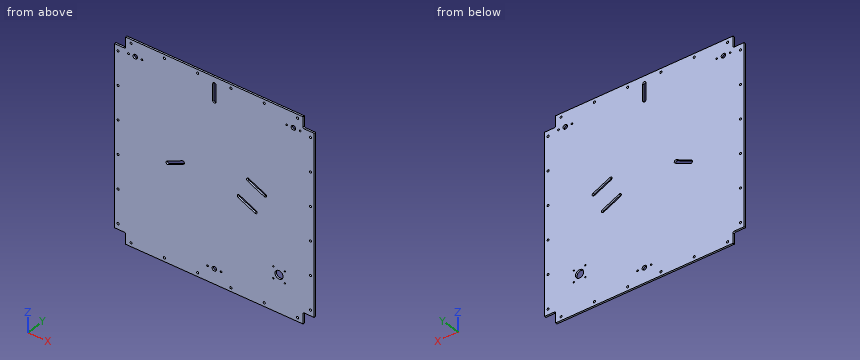
```python
from build123d import *

# Parameters (mm, degrees)
SKETCH2_W             = 540
SKETCH2_H             = 540
SKETCH2_R             = 6
SKETCH2_R_2           = 11
BOSS_EXTRUDE1_DEPTH   = 4.7625
M4_CLEARANCE_HOLE1_D  = 4.5
M3_CLEARANCE_HOLE10_D = 3.4
SKETCH5_W             = 30
SKETCH5_H             = 30
CUT_EXTRUDE1_DEPTH    = 764.6901737
FILLET1_R             = 3.175
CUT_EXTRUDE2_DEPTH    = 764.6901737
CUT_EXTRUDE3_DEPTH    = 764.6901737
M5_CLEARANCE_HOLE1_D  = 5.8
LPATTERN1_COUNT       = 6
LPATTERN1_PITCH       = 90
M5_CLEARANCE_HOLE2_D  = 5.8
LPATTERN2_COUNT       = 6
LPATTERN2_PITCH       = 90
M5_CLEARANCE_HOLE3_D  = 5.8
LPATTERN3_COUNT       = 6
LPATTERN3_PITCH       = 90
M5_CLEARANCE_HOLE4_D  = 5.8
LPATTERN4_COUNT       = 6
LPATTERN4_PITCH       = 90


with BuildPart() as part:
    # Sketch2 → Boss-Extrude1 (new body)
    with BuildSketch(Plane(origin=(0, 0, 0), x_dir=(1, 0, 0), z_dir=(0, 1, 0))):
        with Locations((270, 270)):
            Rectangle(SKETCH2_W, SKETCH2_H)
        with Locations(Location((56.175, 40, 0), (0, 0, 90))):
            Circle(SKETCH2_R, mode=Mode.SUBTRACT)
        with Locations(Location((483.825, 40, 0), (0, 0, 90))):
            Circle(SKETCH2_R, mode=Mode.SUBTRACT)
        with Locations(Location((270, 500, 0), (0, 0, 90))):
            Circle(SKETCH2_R, mode=Mode.SUBTRACT)
        with Locations(Location((445, 440, 0), (0, 0, 90))):
            Circle(SKETCH2_R_2, mode=Mode.SUBTRACT)
    extrude(amount=BOSS_EXTRUDE1_DEPTH)

    # M4 Clearance Hole1 (through all)
    with Locations(Plane(origin=(74.425, 4.7625, -40), x_dir=(0, 0, 1), z_dir=(0, 1, 0))):
        with Locations((0, 0), (0, -36.5), (-460, 177.325), (-460, 213.825), (0, 391.15), (0, 427.65)):
            Hole(M4_CLEARANCE_HOLE1_D / 2)

    # M3 Clearance Hole10 (through all)
    with Locations(Plane(origin=(429.5, 4.7625, -455.5), x_dir=(0, 0, 1), z_dir=(0, 1, 0))):
        with Locations((0, 0), (0, 31), (31, 31), (31, 0)):
            Hole(M3_CLEARANCE_HOLE10_D / 2)

    # Sketch5 → Cut-Extrude1 (cut, through all)
    with BuildSketch(Plane(origin=(0, 4.7625, 0), x_dir=(1, 0, 0), z_dir=(0, 1, 0))):
        with Locations((15, 15)):
            Rectangle(SKETCH5_W, SKETCH5_H)
        with Locations((525, 15)):
            Rectangle(SKETCH5_W, SKETCH5_H)
        with Locations((525, 525)):
            Rectangle(SKETCH5_W, SKETCH5_H)
        with Locations((15, 525)):
            Rectangle(SKETCH5_W, SKETCH5_H)
    extrude(amount=-CUT_EXTRUDE1_DEPTH, mode=Mode.SUBTRACT)

    # Fillet1
    fillet1_edges = [part.edges().sort_by_distance(p)[0] for p in [
        (510, 2.38125, -30),
        (510, 2.38125, -510),
        (30, 2.38125, -510),
        (30, 2.38125, -30),
    ]]
    fillet(fillet1_edges, radius=FILLET1_R)

    # Sketch6 → Cut-Extrude2 (cut, through all)
    with BuildSketch(Plane(origin=(0, 4.7625, 0), x_dir=(1, 0, 0), z_dir=(0, 1, 0))):
        with BuildLine():
            Line((379.893699129, 307.475094097), (334.552801834, 286.398969393))
            ThreePointArc((334.552801834, 286.398969393), (332.490296164, 280.753522523), (338.135743034, 278.691016853))
            Line((338.135743034, 278.691016853), (383.476640328, 299.767141557))
            ThreePointArc((383.476640328, 299.767141557), (385.539145999, 305.412588427), (379.893699129, 307.475094097))
        make_face()
        with BuildLine():
            Line((405.008613589, 253.445580936), (359.667716294, 232.369456232))
            ThreePointArc((359.667716294, 232.369456232), (357.605210624, 226.724009362), (363.250657494, 224.661503692))
            Line((363.250657494, 224.661503692), (408.591554788, 245.737628396))
            ThreePointArc((408.591554788, 245.737628396), (410.654060459, 251.383075266), (405.008613589, 253.445580936))
        make_face()
    extrude(amount=-CUT_EXTRUDE2_DEPTH, mode=Mode.SUBTRACT)

    # Sketch9 → Cut-Extrude3 (cut, through all)
    with BuildSketch(Plane(origin=(0, 4.7625, 0), x_dir=(1, 0, 0), z_dir=(0, 1, 0))):
        with BuildLine():
            Line((274.25, 19), (274.25, 64))
            ThreePointArc((274.25, 64), (270, 68.25), (265.75, 64))
            Line((265.75, 64), (265.75, 19))
            ThreePointArc((265.75, 19), (270, 14.75), (274.25, 19))
        make_face()
        with BuildLine():
            Line((186.642601301, 263.737436412), (145.835793736, 282.705948646))
            ThreePointArc((145.835793736, 282.705948646), (140.190346866, 280.643442976), (142.252852537, 274.997996106))
            Line((142.252852537, 274.997996106), (183.059660101, 256.029483872))
            ThreePointArc((183.059660101, 256.029483872), (188.705106971, 258.091989542), (186.642601301, 263.737436412))
        make_face()
    extrude(amount=-CUT_EXTRUDE3_DEPTH, mode=Mode.SUBTRACT)

    # M5 Clearance Hole1 (through all)
    with Locations(Plane(origin=(45, 4.7625, -10), x_dir=(0, 0, 1), z_dir=(0, 1, 0))):
        with Locations((0, 0)):
            m5_clearance_hole1 = Hole(M5_CLEARANCE_HOLE1_D / 2)

    # LPattern1: M5 Clearance Hole1 ×6
    with Locations(*[(i * LPATTERN1_PITCH, 0, 0) for i in range(1, LPATTERN1_COUNT)]):
        add(m5_clearance_hole1, mode=Mode.SUBTRACT)

    # M5 Clearance Hole2 (through all)
    with Locations(Plane(origin=(10, 4.7625, -495), x_dir=(0, 0, 1), z_dir=(0, 1, 0))):
        with Locations((0, 0)):
            m5_clearance_hole2 = Hole(M5_CLEARANCE_HOLE2_D / 2)

    # LPattern2: M5 Clearance Hole2 ×6
    with Locations(*[(0, 0, i * LPATTERN2_PITCH) for i in range(1, LPATTERN2_COUNT)]):
        add(m5_clearance_hole2, mode=Mode.SUBTRACT)

    # M5 Clearance Hole3 (through all)
    with Locations(Plane(origin=(495, 4.7625, -530), x_dir=(0, 0, 1), z_dir=(0, 1, 0))):
        with Locations((0, 0)):
            m5_clearance_hole3 = Hole(M5_CLEARANCE_HOLE3_D / 2)

    # LPattern3: M5 Clearance Hole3 ×6
    with Locations(*[(-i * LPATTERN3_PITCH, 0, 0) for i in range(1, LPATTERN3_COUNT)]):
        add(m5_clearance_hole3, mode=Mode.SUBTRACT)

    # M5 Clearance Hole4 (through all)
    with Locations(Plane(origin=(530, 4.7625, -45), x_dir=(0, 0, 1), z_dir=(0, 1, 0))):
        with Locations((0, 0)):
            m5_clearance_hole4 = Hole(M5_CLEARANCE_HOLE4_D / 2)

    # LPattern4: M5 Clearance Hole4 ×6
    with Locations(*[(0, 0, -i * LPATTERN4_PITCH) for i in range(1, LPATTERN4_COUNT)]):
        add(m5_clearance_hole4, mode=Mode.SUBTRACT)


solid = part.part
```
Read the model definition and answer for the solid it produces. Units are mm, in the model's axes. Coordinates: 2 decimals unless noted, no trailing zeros. Write each loop counter-clockwise with the first axis right and the second up, starting at its lowest first coordinate (ties: lowest second). Pieces come first, ordered by that corner, then holes. Notation, with made-up numbers: (84.5, 11.25) - (102.5, 11.25) arc R13 cw to (102.5, 20.25) - close; hole circle Ø11 at (19, 35.25). An arc over 180 degrees is marked (long way). Answer as a JSON object with one key per item and string values. Group by question number.
1. A cutting plane is placed at A-A (x = 166). Determine the outline of the cut face in (y, z), plus the area to 3 significant figures.
2. This flat-tipped pin is pushed along its axis until it touches: P1, Ø1.4, axis at x = 13.5, y = 1.5, coming from the -Z side. Where does it stop, or does it pass through?
3. Consider L1, parallel to X at y = 3.15, z = -315; L2, parallel to X at y = 3.65, z = -424.5; L3, parallel to Z at x = 405, y = 3.35. Determine where each line is inside the solid, lowest interval first. Write a range as [from, to].
4. A cutting plane is placed at B-B (y = 2.05). Give the number of separate pieces and of enclosed holes in the cut face, plus the area to 3 significant figures.
Worked out:
{
 "1": {"outline": "(0, -540) - (4.76, -540) - (4.76, -273.33) - (0, -273.33) - close; (0, -263.96) - (4.76, -263.96) - (4.76, 0) - (0, 0) - close", "area": "2,530 mm²"},
 "2": {"P1": "stops at z = -510"},
 "3": {"L1": "x = [0, 7.1], [12.9, 527.1], [532.9, 540]", "L2": "x = [0, 427.8], [431.2, 458.8], [462.2, 540]", "L3": "z = [-540, -532.9], [-527.1, -253.44], [-244.07, -12.9], [-7.1, 0]"},
 "4": {"separate pieces": "1", "enclosed holes": "42", "area": "285,000 mm²"}
}
